Geometry check sheet. Reference: the model listing, model coordinates, mm. Round coordinates to 2 decimals unless told otherwise and drop trailing zeros. Order: outer loops, then holes, each group sorted by start corner. A loop starts at its lowest first (then second) coordinate and runs counter-clockwise, first axis right, second up. Notation, with made-up numbers: M 60.5,39 L 114.5,39 A15 cw 114.5,49 Z; hole C 88,49.5 d8. An arc over 180 degrees is marked long. Return JSON: item names as keys, results as strings. Group by question number.
```python
from build123d import *

# Parameters (mm, degrees)
BOSS_EXTRUDE1_DEPTH  = 5
BOSS_EXTRUDE2_DEPTH  = 5
M5_CLEARANCE_HOLE1_D = 5.5


with BuildPart() as part:
    # Sketch1 → Boss-Extrude1 (new body)
    with BuildSketch(Plane.XY):
        Polygon((0, 0), (20, 0), (230, 122), (210, 122), align=None)
    extrude(amount=BOSS_EXTRUDE1_DEPTH)

    # Sketch2 → Boss-Extrude2 (add)
    with BuildSketch(Plane.XY.offset(5)):
        Polygon((0, 0), (0, 30), (200, 122), (210, 122), (230, 122), (230, 92), (30, 0), align=None)
    extrude(amount=-BOSS_EXTRUDE2_DEPTH)

    # M5 Clearance Hole1 (through all)
    with Locations(Plane.XY.offset(5)):
        with Locations((10, 25), (220, 97), (10, 12.5), (220, 109.5)):
            Hole(M5_CLEARANCE_HOLE1_D / 2)


solid = part.part
```
Q1. Section check B-B on z = 0.75. Record the cut outline in (x, y).
Q2. Section check D-D on x = 130. Record the cut outline in (y, z), plus the area to 3 significant figures.
Q3. Depth check by flat-ended pin: pin 1 Ø1.5 at (x, y) = (153, 84.5) entering from -Z; pin 2 Ø3 at (y, z) = (38, 1.5) entering from +X; pin 3 Ø3.5 at (x, y) = (10, 12.5) entering from -Z; pin 4 Ø3 at (y, z) = (64, 2) entering from +X. Enter the tip coordinate at first touch or a pass-through.
Q4. Section check A-A on x = 220. Record the cut outline in (y, z).
Q5. Section check C-C on y = 97. Record the cut outline in (x, z), plus the area to 3 significant figures.
Q6. Material ranges on line 1 along Y through (x, z) = (220, 3.35); line 2 along Y through (x, z) = (10, 3.3); line 3 along Y through (x, z) = (89, 2), recorded low to high.
Q7. Release check for a two-part mould opening along Y. For faces 1 (the face through (0, 15, 3)), 2 (the face through (215, 122, 3)), 3 (the face through (10.358, 27.727, 2.465)), 4 (the face through (217.46, 108.45, 2.46)) record: +Y half, -Y half, draft (parallel to the pull), parting line (faces both ways), or undercut.
Geometry check:
{
 "1": {"outline": "M 0,0 L 30,0 L 230,92 L 230,122 L 200,122 L 0,30 Z; hole C 10,12.5 d5.5; hole C 10,25 d5.5; hole C 220,97 d5.5; hole C 220,109.5 d5.5"},
 "2": {"outline": "M 46,0 L 89.8,0 L 89.8,5 L 46,5 Z", "area": "219 mm^2"},
 "3": {"pin 1": "stops at z = 0", "pin 2": "stops at x = 115.87", "pin 3": "passes through", "pin 4": "stops at x = 172.39"},
 "4": {"outline": "M 87.4,0 L 94.25,0 L 94.25,5 L 87.4,5 Z; M 99.75,0 L 106.75,0 L 106.75,5 L 99.75,5 Z; M 112.25,0 L 122,0 L 122,5 L 112.25,5 Z"},
 "5": {"outline": "M 145.65,0 L 217.25,0 L 217.25,5 L 145.65,5 Z; M 222.75,0 L 230,0 L 230,5 L 222.75,5 Z", "area": "394 mm^2"},
 "6": {"line 1": "y = 87.4 to 94.25, 99.75 to 106.75, 112.25 to 122", "line 2": "y = 0 to 9.75, 15.25 to 22.25, 27.75 to 34.6", "line 3": "y = 27.14 to 70.94"},
 "7": {"face 1": "draft", "face 2": "+Y half", "face 3": "undercut", "face 4": "undercut"}
}
